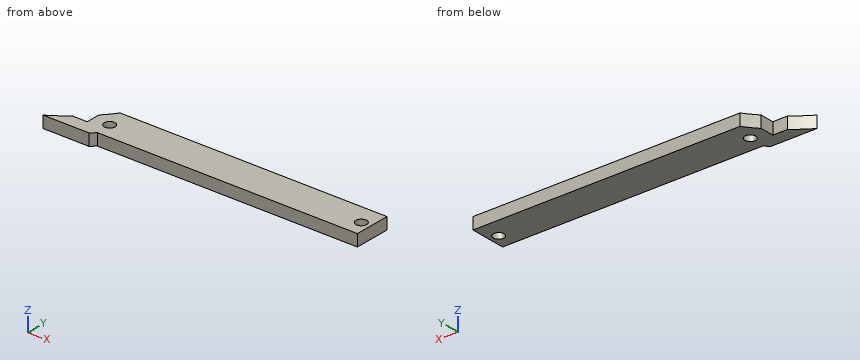
```python
from build123d import *

# Parameters (mm, degrees)
SKETCH1_R           = 1.47
BOSS_EXTRUDE1_DEPTH = 3.18
SKETCH3_R           = 1.47
CUT_EXTRUDE1_DEPTH  = 76.165537316
CUT_EXTRUDE2_START  = -0.08
SKETCH4_W           = 75
SKETCH4_H           = 3.18
CUT_EXTRUDE2_DEPTH  = 0.08
BOSS_EXTRUDE2_DEPTH = 3.18


with BuildPart() as part:
    # Sketch1 → Boss-Extrude1 (new body)
    with BuildSketch(Plane.XY):
        with BuildLine():
            Line((0, 0), (0, 3.84))
            Line((0, 3.84), (75, 3.84))
            Line((75, 3.84), (75, 0.02441688))
            Line((75, 0.02441688), (75, -2.47558312))
            Line((75, -2.47558312), (4.70169557, -2.47558312))
            Line((4.70169557, -2.47558312), (3.5, -3.67727869))
            Line((3.5, -3.67727869), (-9, -3.67727869))
            ThreePointArc((-9, -3.67727869), (-6.432825468, -1.973348375), (-4, -0.082548586))
            Line((-4, -0.082548586), (0, -0.082548586))
            Line((0, -0.082548586), (0, 0))
        make_face()
        with Locations(Location((72.5, 1.84, 0), (0, 0, 180))):
            Circle(SKETCH1_R, mode=Mode.SUBTRACT)
    extrude(amount=BOSS_EXTRUDE1_DEPTH)

    # Sketch3 → Cut-Extrude1 (cut, through all)
    with BuildSketch(Plane.XY.offset(3.18)):
        with Locations((4.5, 1.84)):
            Circle(SKETCH3_R)
    extrude(amount=-CUT_EXTRUDE1_DEPTH, mode=Mode.SUBTRACT)

    # Sketch4 → Cut-Extrude2 (cut)
    with BuildSketch(Plane(origin=(0, 3.84, 0), x_dir=(1, 0, 0), z_dir=(0, 1, 0)).offset(CUT_EXTRUDE2_START)):
        with Locations((37.5, -1.59)):
            Rectangle(SKETCH4_W, SKETCH4_H)
    extrude(amount=CUT_EXTRUDE2_DEPTH, mode=Mode.SUBTRACT)

    # Sketch6 → Boss-Extrude2 (add)
    with BuildSketch(Plane(origin=(0, 0, 0), x_dir=(-1, 0, 0), z_dir=(0, 0, -1))):
        with BuildLine():
            Line((-2.850337408, 7.26), (-75, 7.26))
            Line((-75, 7.26), (-75, 3.76))
            Line((-75, 3.76), (0, 3.76))
            ThreePointArc((0, 3.76), (-1.47307826, 5.470983314), (-2.850337408, 7.26))
        make_face()
    extrude(amount=-BOSS_EXTRUDE2_DEPTH)


solid = part.part
```
The model under review builds one solid part; all positions refer to its coordinate system, in mm. Give positions to 0.01 mm unless a question says otherwise; leave off trailing zeros. Write each loop counter-clockwise with the first axis right and the second up, starting at its lowest first coordinate (ties: lowest second). Pieces come first, ordered by that corner, then holes.
(1) To check wall thickness, follow L1, parallel to X at y = 2.5, z = 1.15; L2, parallel to Y at x = 72.5, z = 2.4; L3, parallel to Y at x = 34, z = 0.2. State the ranges of each line that lie inside material, in increasing order.
(2) Consider section A-A, the plane x = 72.5. Give the boundary of the cut face in (y, z).
(3) Consider section C-C, the plane z = 1.2. Give the boundary of the cut face in (x, y), and give its area (3 significant figures).
(4) For P1, Ø1.5, axis at x = 29.5, z = 0.5, coming from the -Y side; P2, Ø1.6, axis at y = 2.5, z = 2.5, coming from the -X side, all flat-tipped, find the tip position at first contact; note any pin that passes through.
(5) Consider section D-D, the plane x = 21.5. Give the boundary of the cut face in (y, z).
(6) Consider section B-B, the plane y = 1.84. Give the boundary of the cut face in (x, z), and give its area (3 significant figures).
Returned:
1. L1: x = 0 to 3.19, 5.81 to 71.19, 73.81 to 75
1. L2: y = -2.48 to 0.37, 3.31 to 7.26
1. L3: y = -2.48 to 7.26
2. outline: (-2.48, 0) - (0.37, 0) - (0.37, 3.18) - (-2.48, 3.18) - close; (3.31, 0) - (7.26, 0) - (7.26, 3.18) - (3.31, 3.18) - close
3. outline: (-9, -3.68) - (3.5, -3.68) - (4.7, -2.48) - (75, -2.48) - (75, 7.26) - (2.85, 7.26) arc R41.25 cw to (0, 3.76) - (0, -0.08) - (-4, -0.08) arc R41.25 cw to start; hole circle Ø2.94 at (4.5, 1.84); hole circle Ø2.94 at (72.5, 1.84)
3. area: 739 mm2
4. P1: stops at y = -2.48
4. P2: stops at x = 0
5. outline: (-2.48, 0) - (7.26, 0) - (7.26, 3.18) - (-2.48, 3.18) - close
6. outline: (0, 0) - (3.03, 0) - (3.03, 3.18) - (0, 3.18) - close; (5.97, 0) - (71.03, 0) - (71.03, 3.18) - (5.97, 3.18) - close; (73.97, 0) - (75, 0) - (75, 3.18) - (73.97, 3.18) - close
6. area: 220 mm2
